Work out the finished part from the listing and answer in its coordinate system (mm). Coordinates: 2 decimals unless noted, no trailing zeros. Loops run counter-clockwise (first coordinate to the right, second up) from the corner with the lowest first, then second, coordinate; pieces in that order, holes last. Notation, with made-up numbers: (-12, -27.5) -> (27, -27.5) arc R24 cw to (27, -17.5) -> close; hole circle Ø5 at (-9.5, 81). An arc over 180 degrees is marked (long way). Answer as CSV lines item,"result".
```python
from build123d import *

# Parameters (mm, degrees)
EXTRUDE_1_DEPTH     = 6
SKETCH_2_R          = 1.6
CUT_EXTRUDE_1_DEPTH = 10
SKETCH_3_OUTSIDE_W  = 89.27
SKETCH_3_OUTSIDE_H  = 89.27
CUT_EXTRUDE_2_DEPTH = 10
FILLET_1_R          = 5
FILLET_2_R          = 2


with BuildPart() as part:
    # 草图1 → 凸台-拉伸1 (new body)
    with BuildSketch(Plane(origin=(0, 0, 0), x_dir=(1, 0, 0), z_dir=(0, 1, 0))):
        with BuildLine():
            Line((-20.199009877, 31), (20.199009877, 31))
            ThreePointArc((20.199009877, 31), (26.162950904, 26.162950904), (31, 20.199009877))
            Line((31, 20.199009877), (31, -20.199009877))
            ThreePointArc((31, -20.199009877), (-26.162950904, -26.162950904), (-20.199009877, 31))
        make_face()
    extrude(amount=EXTRUDE_1_DEPTH)

    # 草图2 → 切除-拉伸1 (cut)
    with BuildSketch(Plane(origin=(0, 6, 0), x_dir=(1, 0, 0), z_dir=(0, 1, 0))):
        with Locations(Location((26.998940675, 18.975173317, 0), (0, 0, 270))):
            Circle(SKETCH_2_R)
        with Locations(Location((18.975173317, 26.998940675, 0), (0, 0, 270))):
            Circle(SKETCH_2_R)
    extrude(amount=-CUT_EXTRUDE_1_DEPTH, mode=Mode.SUBTRACT)

    # 草图3 outside → 切除-拉伸2 (cut)
    with BuildSketch(Plane(origin=(0, 6, 0), x_dir=(1, 0, 0), z_dir=(0, 1, 0))):
        with Locations((-3, -3)):
            Rectangle(SKETCH_3_OUTSIDE_W, SKETCH_3_OUTSIDE_H)
        with BuildLine():
            Line((0.691210962, 31), (9.386018717, 23.171159933))
            ThreePointArc((9.386018717, 23.171159933), (17.67766953, 17.67766953), (23.171159933, 9.386018717))
            Line((23.171159933, 9.386018717), (31, 0.691210962))
            Line((31, 0.691210962), (31, 20.199009877))
            ThreePointArc((31, 20.199009877), (26.162950904, 26.162950904), (20.199009877, 31))
            Line((20.199009877, 31), (0.691210962, 31))
        make_face(mode=Mode.SUBTRACT)
    extrude(amount=-CUT_EXTRUDE_2_DEPTH, mode=Mode.SUBTRACT)

    # 圆角1
    fillet_1_edges = [part.edges().sort_by_distance(p)[0] for p in [
        (20.199009877, 3, -31),
        (31, 3, -20.199009877),
    ]]
    fillet(fillet_1_edges, radius=FILLET_1_R)

    # 圆角2
    fillet_2_edges = [part.edges().sort_by_distance(p)[0] for p in [
        (31, 3, -0.691210962),
        (0.691210962, 3, -31),
    ]]
    fillet(fillet_2_edges, radius=FILLET_2_R)


solid = part.part
```
(1) A cutting plane is placed at B-B, the plane y = 2.4. Write down the section's boundary in (x, z).
Computed values:
outline,"(4.56, -27.51) arc R2 ccw to (5.9, -31) -> (18.65, -31) arc R5 ccw to (21.57, -30.06) arc R37 ccw to (30.06, -21.57) arc R5 ccw to (31, -18.65) -> (31, -5.9) arc R2 ccw to (27.51, -4.56) -> (23.17, -9.39) arc R25 cw to (9.39, -23.17) -> close; hole circle Ø3.2 at (18.98, -27); hole circle Ø3.2 at (27, -18.98)"
(2) A cutting plane is placed at D-D, the plane x = 7.75. Write down the section's boundary in (y, z).
Computed values:
outline,"(0, -31) -> (6, -31) -> (6, -24.64) -> (0, -24.64) -> close"
(3) A cutting plane is placed at A-A, the plane z = -27. Write down the section's boundary in (x, y).
Computed values:
outline,"(5.13, 0) -> (17.38, 0) -> (17.38, 6) -> (5.13, 6) -> close; (20.58, 0) -> (25.3, 0) -> (25.3, 6) -> (20.58, 6) -> close"
(4) For a pull along Z with two mould halves and no side action, classify faces 1 (the face through (12, 3, -31)), 2 (the face through (25.6, 3, -18.2)), 3 (the face through (19, 3, -28.6)), 4 (the face through (6.941, 3.042, -25.373)) as pulls with the +Z half, pulls with the -Z half, needs draft (parallel to the pull), parting line crosses it, or undercut.
Computed values:
face 1,"pulls with the -Z half"
face 2,"undercut"
face 3,"undercut"
face 4,"pulls with the +Z half"
(5) A cutting plane is placed at C-C, the plane x = 19.5. Write down the section's boundary in (y, z), and give its area (3 significant figures).
Computed values:
outline,"(0, -30.93) -> (6, -30.93) -> (6, -28.51) -> (0, -28.51) -> close; (0, -25.49) -> (6, -25.49) -> (6, -15.64) -> (0, -15.64) -> close"
area,"73.6 mm2"
(6) Flat-ended cylindrical pins translate along their axes: pin 1 Ø1 at (x, y) = (13, 5) entering from +Z; pin 2 Ø3 at (x, z) = (27, -18.98) entering from -Y; pin 3 Ø2 at (y, z) = (3.5, -23.5) entering from +X. Find the tip coordinate at first contact, or state that the pin passes through.
Computed values:
pin 1,"z = -21.04"
pin 2,"through"
pin 3,"x = 29.37"
(7) Consider line 1 along Z through (x, y) = (26.25, 1.15); line 2 along Z through (x, y) = (27.75, 1.85); line 3 along X through (y, z) = (2, -27.5). Determine where each line is inside the solid, lowest interval first.
Computed values:
line 1,"-26.08 to -20.39, -17.56 to -5.97"
line 2,"-24.47 to -20.39, -17.56 to -4.34"
line 3,"4.58 to 17.46, 20.49 to 24.75"
